Source: CAD feature listing. Evaluate the final solid. Frame: model axes, mm. A direction names the side the tool comes from. Give positions to 0.01 mm unless a question says otherwise; leave off trailing zeros. Order: outer loops, then holes, each group sorted by start corner. A loop starts at its lowest first (then second) coordinate and runs counter-clockwise, first axis right, second up. Notation, with made-up numbers: M 12,59 L 63,59 A23 ccw 63,88 Z; hole C 28.25,-27 d7. An arc over 180 degrees is marked long. Answer in a Markdown table with one row per item. Add a question column.
(1) Section query B-B, the plane y = -9. Return loops of the section in (x, z), plus the area to 3 significant figures.
(2) Pin query (flat end, axial travel): P1, Ø5.5, axis at x = -128, y = -53, coming from the -Z side; P2, Ø1, axis at y = 32.5, z = -6, coming from the +X side; P3, Ø10, axis at x = 129, y = -52, coming from the +Z side; P4, Ø7, axis at x = -128, y = 53, coming from the +Z side. Return the tip coordinate at first contact, or that it passes through.
(3) Section query D-D, the plane x = 57. Return loops of the section in (y, z), plus the area to 4 significant figures.
(4) Section query A-A, the plane z = -4.25. Return loops of the section in (x, y), plus the area to 3 significant figures.
(5) Section query C-C, the plane x = 15. Return loops of the section in (y, z).
(6) Set-up query: faces 1 (the face through (1, -33, -10)), 2 (the face through (130, -51, 1.9)), 3 (the face through (-47.75, -1, -5)), 4 (the face through (1, 27.75, -5)), 5 (the face through (1, 37.75, -5)). Return all of +Z, -Z, +X, -X, +Y, -Y with unobstructed straight access to the full face (end or side cutting, diameter ignored); none if empty.
(7) Material intervals for line 1 along Y through (x, z) = (9, -9); line 2 along X through (y, z) = (18, -4.75); line 3 along X through (y, z) = (-53, 1.25), sorted ascending.
from build123d import *

# Parameters (mm, degrees)
BOSS_EXTRUDE1_DEPTH                           = 5
CBORE_FOR_M4_PAN_HEAD_MACHINE_SCREW1_AT_COUNT = 2
CBORE_FOR_M4_PAN_HEAD_MACHINE_SCREW1_AT_PITCH = 106
CBORE_FOR_M4_PAN_HEAD_MACHINE_SCREW1_2_COUNT  = 2
CBORE_FOR_M4_PAN_HEAD_MACHINE_SCREW1_2_PITCH  = 256
CBORE_FOR_M4_PAN_HEAD_MACHINE_SCREW1_3_COUNT  = 2
CBORE_FOR_M4_PAN_HEAD_MACHINE_SCREW1_3_PITCH  = 277.077606457
SKETCH4_W                                     = 95.5
SKETCH4_H                                     = 75.5
SKETCH4_W_2                                   = 75.5
SKETCH4_H_2                                   = 55.5
BOSS_EXTRUDE2_DEPTH                           = 10


with BuildPart() as part:
    # Sketch1 → Boss-Extrude1 (new body)
    with BuildSketch(Plane.XY):
        with BuildLine():
            Line((-119.75, 64.75), (119.75, 64.75))
            ThreePointArc((119.75, 64.75), (133.892135624, 58.892135624), (139.75, 44.75))
            Line((139.75, 44.75), (139.75, -44.75))
            ThreePointArc((139.75, -44.75), (133.892135624, -58.892135624), (119.75, -64.75))
            Line((119.75, -64.75), (-119.75, -64.75))
            ThreePointArc((-119.75, -64.75), (-133.892135624, -58.892135624), (-139.75, -44.75))
            Line((-139.75, -44.75), (-139.75, 44.75))
            ThreePointArc((-139.75, 44.75), (-133.892135624, 58.892135624), (-119.75, 64.75))
        make_face()
    extrude(amount=BOSS_EXTRUDE1_DEPTH)

    # Sketch3 → CBORE for M4 Pan Head Machine Screw1 (revolve, cut)
    with BuildSketch(Plane(origin=(-128, 53, 5), x_dir=(0, -1, 0), z_dir=(1, 0, 0))):
        Polygon((0, 0), (0, 31.351936393), (2.25, 30), (2.25, 3.1), (4.5, 3.1), (4.5, 0.025), (4.525, 0), align=None)
    cbore_for_m4_pan_head_machine_screw1 = revolve(axis=Axis((-128, 53, 11.35), (0, 0, -1)), mode=Mode.SUBTRACT)

    # CBORE for M4 Pan Head Machine Screw1 at: CBORE for M4 Pan Head Machine Screw1 ×2
    with Locations(*[(0, -i * CBORE_FOR_M4_PAN_HEAD_MACHINE_SCREW1_AT_PITCH, 0) for i in range(1, CBORE_FOR_M4_PAN_HEAD_MACHINE_SCREW1_AT_COUNT)]):
        add(cbore_for_m4_pan_head_machine_screw1, mode=Mode.SUBTRACT)

    # CBORE for M4 Pan Head Machine Screw1 2: CBORE for M4 Pan Head Machine Screw1 ×2
    with Locations(*[(i * CBORE_FOR_M4_PAN_HEAD_MACHINE_SCREW1_2_PITCH, 0, 0) for i in range(1, CBORE_FOR_M4_PAN_HEAD_MACHINE_SCREW1_2_COUNT)]):
        add(cbore_for_m4_pan_head_machine_screw1, mode=Mode.SUBTRACT)

    # CBORE for M4 Pan Head Machine Screw1 3: CBORE for M4 Pan Head Machine Screw1 ×2
    with Locations(*[Vector(0.9239288705910963, -0.38256429797912583, 0) * (i * CBORE_FOR_M4_PAN_HEAD_MACHINE_SCREW1_3_PITCH) for i in range(1, CBORE_FOR_M4_PAN_HEAD_MACHINE_SCREW1_3_COUNT)]):
        add(cbore_for_m4_pan_head_machine_screw1, mode=Mode.SUBTRACT)

    # Sketch4 → Boss-Extrude2 (add)
    with BuildSketch(Plane(origin=(0, 0, 0), x_dir=(-1, 0, 0), z_dir=(0, 0, -1))):
        Rectangle(SKETCH4_W, SKETCH4_H)
        Rectangle(SKETCH4_W_2, SKETCH4_H_2, mode=Mode.SUBTRACT)
    extrude(amount=BOSS_EXTRUDE2_DEPTH)


solid = part.part
Values follow:
| question | item | result |
|---|---|---|
| 1 | outline | M -139.75,0 L -47.75,0 L -47.75,-10 L -37.75,-10 L -37.75,0 L 37.75,0 L 37.75,-10 L 47.75,-10 L 47.75,0 L 139.75,0 L 139.75,5 L -139.75,5 Z |
| 1 | area | 1,600 mm² |
| 2 | P1 | stops at z = 0 |
| 2 | P2 | stops at x = 47.75 |
| 2 | P3 | stops at z = 5 |
| 2 | P4 | stops at z = 1.9 |
| 3 | outline | M -64.75,0 L 64.75,0 L 64.75,5 L -64.75,5 Z |
| 3 | area | 647.5 mm² |
| 4 | outline | M -47.75,-37.75 L 47.75,-37.75 L 47.75,37.75 L -47.75,37.75 Z; hole M -37.75,-27.75 L 37.75,-27.75 L 37.75,27.75 L -37.75,27.75 Z |
| 4 | area | 3,020 mm² |
| 5 | outline | M -64.75,0 L -37.75,0 L -37.75,-10 L -27.75,-10 L -27.75,0 L 27.75,0 L 27.75,-10 L 37.75,-10 L 37.75,0 L 64.75,0 L 64.75,5 L -64.75,5 Z |
| 6 | face 1 | -Z, +X, -X, +Y, -Y |
| 6 | face 2 | +Z |
| 6 | face 3 | -Z, -X, +Y, -Y |
| 6 | face 4 | -Z |
| 6 | face 5 | -Z, +X, -X, +Y |
| 7 | line 1 | y = -37.75 to -27.75, 27.75 to 37.75 |
| 7 | line 2 | x = -47.75 to -37.75, 37.75 to 47.75 |
| 7 | line 3 | x = -137.97 to -130.25, -125.75 to 125.75, 130.25 to 137.97 |
